```python
from build123d import *

# Parameters (mm, degrees)
SKETCH1_W           = 44
SKETCH1_H           = 31
BOSS_EXTRUDE1_DEPTH = 1.5
SKETCH2_R           = 2.6
SKETCH2_R_2         = 3
CUT_EXTRUDE1_DEPTH  = 1.5


with BuildPart() as part:
    # Sketch1 → Boss-Extrude1 (new body)
    with BuildSketch(Plane(origin=(0, 0, 0), x_dir=(1, 0, 0), z_dir=(0, 1, 0))):
        Rectangle(SKETCH1_W, SKETCH1_H)
    extrude(amount=BOSS_EXTRUDE1_DEPTH)

    # Sketch2 → Cut-Extrude1 (cut)
    with BuildSketch(Plane(origin=(0, 1.5, 0), x_dir=(1, 0, 0), z_dir=(0, 1, 0))):
        with Locations((-17, 10.5)):
            Circle(SKETCH2_R)
        with Locations((17, 10.5)):
            Circle(SKETCH2_R)
        with Locations((17, -10.5)):
            Circle(SKETCH2_R)
        with Locations((-17, -10.5)):
            Circle(SKETCH2_R)
        Circle(SKETCH2_R_2)
    extrude(amount=-CUT_EXTRUDE1_DEPTH, mode=Mode.SUBTRACT)


solid = part.part
```
Source: CAD feature listing. Evaluate the final solid. Frame: model axes, mm. Coordinates: 2 decimals unless noted, no trailing zeros. Loops run counter-clockwise (first coordinate to the right, second up) from the corner with the lowest first, then second, coordinate; pieces in that order, holes last. Notation, with made-up numbers: M 85.25,35 L 97.25,35 A18 ccw 97.25,61 Z; hole C 38,-15.5 d11. An arc over 180 degrees is marked long. Use a Markdown table: item, result. Add a question column.
Q1. Material intervals for L1, parallel to Z at x = 17, y = 0.9; L2, parallel to X at y = 0.55, z = -11; L3, parallel to X at y = 0.35, z = 0, sorted ascending.
Q2. Section query A-A, the plane x = 0. Return loops of the section in (y, z), and give its area (3 significant figures).
Q3. First-contact query: pin 1 (4.5 mm diameter, centred on x = -17, z = 10.5, fed in from -Y). Flat tip, straight axial feed; report the tip coordinate or a pass-through.
Q4. Section query D-D, the plane x = 17. Return loops of the section in (y, z), and give its area (3 significant figures).
Q5. Draft query along Z for faces 1 (the cylindrical face through (19.4, 0.8, 11.5)), 2 (the flat face through (0, 1, 15.5)), 3 (the flat face through (-22, 1, 0)), 4 (the flat face through (0, 1, -15.5)). Return one class per face: pulls with the +Z half, pulls with the -Z half, needs draft (parallel to the pull), parting line crosses it, or undercut.
Q6. Section query B-B, the plane z = 10.5. Return loops of the section in (x, y), and give its area (3 significant figures).
Q7. Section query C-C, the plane y = 0.85. Return loops of the section in (x, z), and give its area (3 significant figures).
Result:
| question | item | result |
|---|---|---|
| 1 | L1 | z = -15.5 to -13.1, -7.9 to 7.9, 13.1 to 15.5 |
| 1 | L2 | x = -22 to -19.55, -14.45 to 14.45, 19.55 to 22 |
| 1 | L3 | x = -22 to -3, 3 to 22 |
| 2 | outline | M 0,-15.5 L 1.5,-15.5 L 1.5,-3 L 0,-3 Z; M 0,3 L 1.5,3 L 1.5,15.5 L 0,15.5 Z |
| 2 | area | 37.5 mm2 |
| 3 | pin 1 | passes through |
| 4 | outline | M 0,-15.5 L 1.5,-15.5 L 1.5,-13.1 L 0,-13.1 Z; M 0,-7.9 L 1.5,-7.9 L 1.5,7.9 L 0,7.9 Z; M 0,13.1 L 1.5,13.1 L 1.5,15.5 L 0,15.5 Z |
| 4 | area | 30.9 mm2 |
| 5 | face 1 | undercut |
| 5 | face 2 | pulls with the +Z half |
| 5 | face 3 | needs draft |
| 5 | face 4 | pulls with the -Z half |
| 6 | outline | M -22,0 L -19.6,0 L -19.6,1.5 L -22,1.5 Z; M -14.4,0 L 14.4,0 L 14.4,1.5 L -14.4,1.5 Z; M 19.6,0 L 22,0 L 22,1.5 L 19.6,1.5 Z |
| 6 | area | 50.4 mm2 |
| 7 | outline | M -22,-15.5 L 22,-15.5 L 22,15.5 L -22,15.5 Z; hole C -17,-10.5 d5.2; hole C -17,10.5 d5.2; hole C 0,0 d6; hole C 17,-10.5 d5.2; hole C 17,10.5 d5.2 |
| 7 | area | 1,250 mm2 |
